Part print with two shaded views. Sizes in mm from the minimum x, y, z corner. Give positions to 0.01 mm unless a question says otherwise; leave off trailing zeros. Order: outer loops, then holes, each group sorted by start corner. A loop starts at its lowest first (then second) coordinate and runs counter-clockwise, first axis right, second up. Notation, with made-up numbers: M 47,-36.5 L 90,-36.5 A17 ccw 90,-23.5 Z; hole C 26,24 d8. An arc over 180 degrees is marked long. Return JSON: item names as keys, results as strings. Group by question number.
1. Slice it at B-B on x = 12. List the corners of the cut face in (y, z) (3 decimals), then the cut area to 3 significant figures.
2. Wall check: probe 1 along Z at (x, y) = (19.05, 2); probe 2 along Y at (x, z) = (27, 30.5) (3 decimals); probe 3 along Z at (x, y) = (36, 11.5) (3 decimals). Give the ranges that are in metal, low to high. Write a range as [from, to].
3. Slice it at A-A on x = 19.05. List the corners of the cut face in (y, z) (1 decimal).
4. Slice it at D-D on z = 3. List the corners of the cut face in (x, y) (3 decimals).
5. Pin check, flat tips, straight feed: pin 1 (10.5 mm diameter, centred on x = 28, z = 23, fed in from +Y) (3 decimals); pin 2 (5.5 mm diameter, centred on x = 23.5, y = 16.5, fed in from -Z) (3 decimals). Stop position of each tip, or through.
6. Slice it at C-C on y = 18.25. List the corners of the cut face in (x, z) (3 decimals), then the cut area to 3 significant figures.
7. Two-plate mould, pull along Z, no slides. Class the marked faces 1, 2 and 3: released by +Z, released by -Z, zero draft, split by the parting line, or undercut.
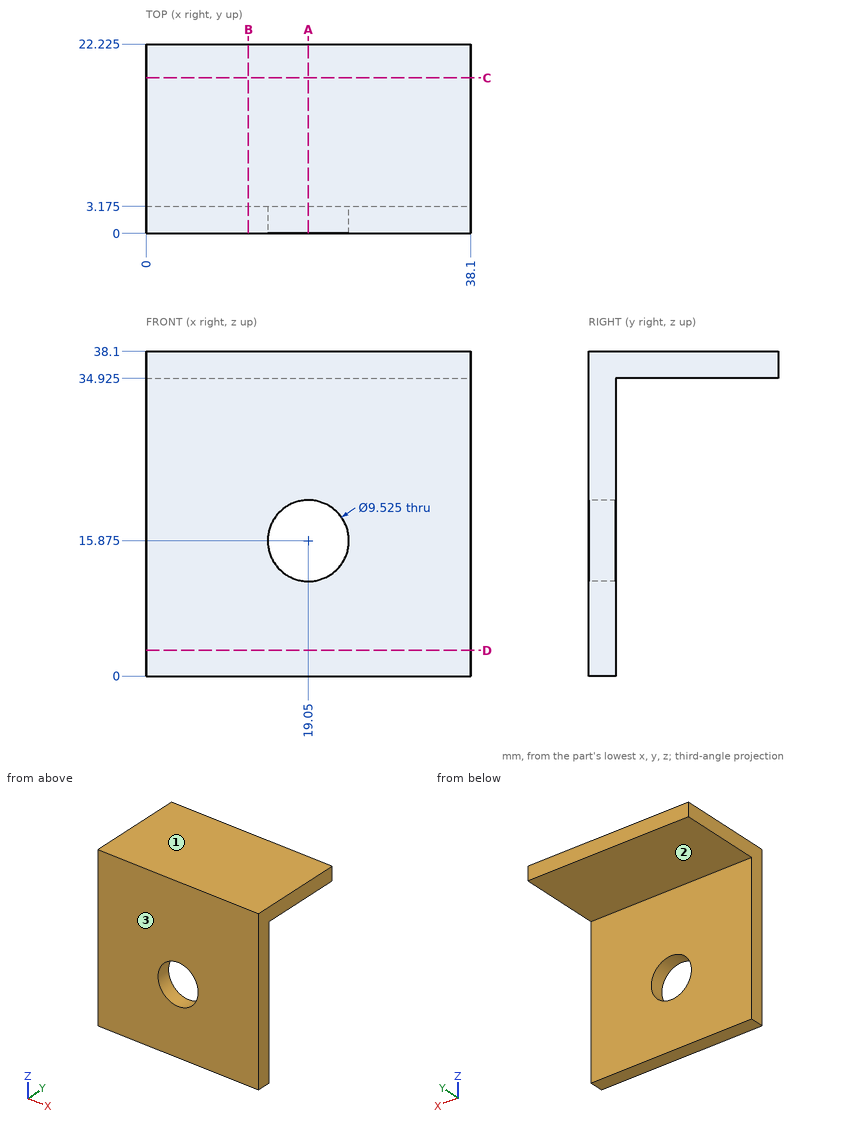
Result:
{
 "1": {"outline": "M 0,0 L 3.175,0 L 3.175,34.925 L 22.225,34.925 L 22.225,38.1 L 0,38.1 Z", "area": "181 mm2"},
 "2": {"probe 1": "z = [0, 11.11], [20.64, 38.1]", "probe 2": "y = [0, 3.175]", "probe 3": "z = [34.925, 38.1]"},
 "3": {"outline": "M 0,0 L 3.2,0 L 3.2,11.1 L 0,11.1 Z; M 0,20.6 L 3.2,20.6 L 3.2,34.9 L 22.2,34.9 L 22.2,38.1 L 0,38.1 Z"},
 "4": {"outline": "M 0,0 L 38.1,0 L 38.1,3.175 L 0,3.175 Z"},
 "5": {"pin 1": "stops at y = 3.175", "pin 2": "stops at z = 34.925"},
 "6": {"outline": "M 0,34.925 L 38.1,34.925 L 38.1,38.1 L 0,38.1 Z", "area": "121 mm2"},
 "7": {"face 1": "released by +Z", "face 2": "released by -Z", "face 3": "zero draft"}
}
